Check sheet for the modelled part. Datum: model origin and axes. Units: mm. Face numbers are marked on the shaded views. Give positions to 0.01 mm unless a question says otherwise; leave off trailing zeros. Write each loop counter-clockwise with the first axis right and the second up, starting at its lowest first coordinate (ties: lowest second). Pieces come first, ordered by that corner, then holes. Notation, with made-up numbers: M 80.5,0 L 106.5,0 A9 cw 106.5,6 Z; hole C -22,35 d3. An arc over 180 degrees is marked long. Write item = value, one per line. Start each with the question number.
1) Cross-section at B-B, the plane y = 13.85. Record the cut outline in (x, z).
2) Cross-section at D-D, the plane y = -5. Record the cut outline in (x, z).
3) Mould release check, pull along X, two halves, no side actions. Record for the marked faces 1 and 2: released by +X, released by -X, zero draft, split by the parting line, or undercut.
4) Cross-section at A-A, the plane x = 0. Record the cut outline in (y, z).
5) Go/stop test with flat-tipped pins: pin 1 (2 mm diameter, centred on x = -33, y = -7, fed in from +Z); pin 2 (1.2 mm diameter, centred on x = 13, z = 3.5, fed in from -Y); pin 3 (2 mm diameter, centred on y = -1.5, z = 4, fed in from +X). Record where each tip stops, or that it passes through.
6) Scan lines: line 1 along Y through (x, z) = (0, 1.6); line 2 along Y through (x, z) = (33, 4); line 3 along X through (y, z) = (2, 2.95). Record each from-to range of solid material in increasing order. Write a range as [from, to].
7) Cross-section at C-C, the plane x = -30.5. Record the cut outline in (y, z).
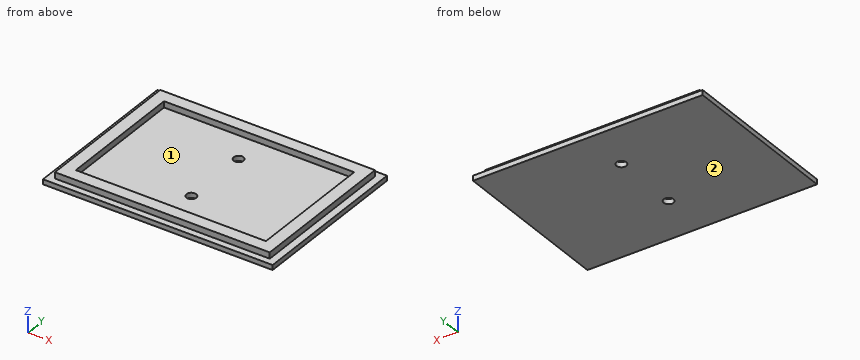
```python
from build123d import *

# Parameters (mm, degrees)
F0_W     = 93
F0_H     = 67
F1_DEPTH = 2
F2_W     = 87
F2_H     = 61.7
F3_DEPTH = 2.5
F4_R     = 2
F5_DEPTH = 4.501
F6_W     = 77
F6_H     = 51.7
F7_DEPTH = 2.5


with BuildPart() as f1:
    # F0 (on Top) → F1 (new body)
    with BuildSketch(Plane.XY):
        Rectangle(F0_W, F0_H)
    extrude(amount=F1_DEPTH)

    # F2 (on face) → F3 (join)
    with BuildSketch(Plane.XY.offset(2)):
        Rectangle(F2_W, F2_H)
    extrude(amount=F3_DEPTH)

    # F4 (on face) → F5 (cut, through all)
    with BuildSketch(Plane.XY.offset(4.5)):
        with Locations((0, 13.85)):
            Circle(F4_R)
        with Locations((0, -13.85)):
            Circle(F4_R)
    extrude(amount=-F5_DEPTH, mode=Mode.SUBTRACT)

    # F6 (on face) → F7 (cut)
    with BuildSketch(Plane.XY.offset(4.5)):
        Rectangle(F6_W, F6_H)
    extrude(amount=-F7_DEPTH, mode=Mode.SUBTRACT)


solid = f1.part
```
Reply:
q1.outline = M -46.5,0 L -2,0 L -2,2 L -38.5,2 L -38.5,4.5 L -43.5,4.5 L -43.5,2 L -46.5,2 Z; M 2,0 L 46.5,0 L 46.5,2 L 43.5,2 L 43.5,4.5 L 38.5,4.5 L 38.5,2 L 2,2 Z
q2.outline = M -46.5,0 L 46.5,0 L 46.5,2 L 43.5,2 L 43.5,4.5 L 38.5,4.5 L 38.5,2 L -38.5,2 L -38.5,4.5 L -43.5,4.5 L -43.5,2 L -46.5,2 Z
q3.face_1 = undercut
q3.face_2 = zero draft
q4.outline = M -33.5,0 L -15.85,0 L -15.85,2 L -25.85,2 L -25.85,4.5 L -30.85,4.5 L -30.85,2 L -33.5,2 Z; M -11.85,0 L 11.85,0 L 11.85,2 L -11.85,2 Z; M 15.85,0 L 33.5,0 L 33.5,2 L 30.85,2 L 30.85,4.5 L 25.85,4.5 L 25.85,2 L 15.85,2 Z
q5.pin_1 = 2
q5.pin_2 = -30.85
q5.pin_3 = 43.5
q6.line_1 = [-33.5, -15.85], [-11.85, 11.85], [15.85, 33.5]
q6.line_2 = [-30.85, -25.85], [25.85, 30.85]
q6.line_3 = [-43.5, -38.5], [38.5, 43.5]
q7.outline = M -33.5,0 L 33.5,0 L 33.5,2 L 30.85,2 L 30.85,4.5 L 25.85,4.5 L 25.85,2 L -25.85,2 L -25.85,4.5 L -30.85,4.5 L -30.85,2 L -33.5,2 Z
